from build123d import *

# Parameters (mm, degrees)
SKETCH1_W                    = 139.7
SKETCH1_H                    = 139.7
BOSS_EXTRUDE1_DEPTH          = 4.064
BOSS_EXTRUDE2_DEPTH          = 24.892
FILLET1_R                    = 4
FILLET2_R                    = 4
F_6_0_6_DIAMETER_HOLE1_D     = 6
F_6_0_6_DIAMETER_HOLE1_DEPTH = 18.75
F_6_0_6_DIAMETER_HOLE1_TIP   = 1.802581857


with BuildPart() as part:
    # Sketch1 → Boss-Extrude1 (new body)
    with BuildSketch(Plane(origin=(0, 0, 0), x_dir=(1, 0, 0), z_dir=(0, 1, 0))):
        Rectangle(SKETCH1_W, SKETCH1_H)
    extrude(amount=BOSS_EXTRUDE1_DEPTH)

    # Sketch2 → Boss-Extrude2 (add)
    with BuildSketch(Plane(origin=(0, 4.064, 0), x_dir=(1, 0, 0), z_dir=(0, 1, 0))):
        Polygon((27.6987, 69.85), (-27.6987, 69.85), (-27.6987, 56.261), (-48.5013, 56.261), (-48.5013, 69.85), (-69.85, 69.85), (-69.85, -69.85), (-48.5013, -69.85), (-48.5013, -56.261), (-27.6987, -56.261), (-27.6987, -69.85), (27.6987, -69.85), (27.6987, -56.261), (48.5013, -56.261), (48.5013, -69.85), (69.85, -69.85), (69.85, 69.85), (48.5013, 69.85), (48.5013, 56.261), (27.6987, 56.261), align=None)
    extrude(amount=BOSS_EXTRUDE2_DEPTH)

    # Fillet1
    fillet1_edges = [part.edges().sort_by_distance(p)[0] for p in [
        (48.5013, 16.51, 69.85),
        (48.5013, 16.51, -69.85),
        (48.5013, 16.51, -56.261),
        (27.6987, 16.51, -56.261),
        (27.6987, 16.51, -69.85),
        (-27.6987, 16.51, -69.85),
        (-27.6987, 16.51, -56.261),
        (-48.5013, 16.51, -56.261),
        (-48.5013, 16.51, -69.85),
        (-48.5013, 16.51, 69.85),
        (-48.5013, 16.51, 56.261),
        (-27.6987, 16.51, 56.261),
        (-27.6987, 16.51, 69.85),
        (27.6987, 16.51, 69.85),
        (27.6987, 16.51, 56.261),
        (48.5013, 16.51, 56.261),
        (69.85, 14.478, 69.85),
        (-69.85, 14.478, 69.85),
        (-69.85, 14.478, -69.85),
        (69.85, 14.478, -69.85),
    ]]
    fillet(fillet1_edges, radius=FILLET1_R)

    # Fillet2
    fillet2_edges = [part.edges().sort_by_distance(p)[0] for p in [
        (47.329727125, 28.956, -57.432572875),
        (28.870272875, 28.956, -57.432572875),
        (-28.870272875, 28.956, -57.432572875),
        (-47.329727125, 28.956, -57.432572875),
        (-47.329727125, 28.956, 57.432572875),
        (-28.870272875, 28.956, 57.432572875),
        (47.329727125, 28.956, 57.432572875),
        (28.870272875, 28.956, 57.432572875),
        (-59.17565, 28.956, -69.85),
        (0, 28.956, -69.85),
        (59.17565, 28.956, -69.85),
        (69.85, 28.956, 0),
        (59.17565, 28.956, 69.85),
        (48.5013, 28.956, -63.0555),
        (38.1, 28.956, -56.261),
        (27.6987, 28.956, -63.0555),
        (-27.6987, 28.956, -63.0555),
        (-38.1, 28.956, -56.261),
        (-48.5013, 28.956, -63.0555),
        (-69.85, 28.956, 0),
        (-59.17565, 28.956, 69.85),
        (-48.5013, 28.956, 63.0555),
        (-38.1, 28.956, 56.261),
        (-27.6987, 28.956, 63.0555),
        (0, 28.956, 69.85),
        (27.6987, 28.956, 63.0555),
        (38.1, 28.956, 56.261),
        (48.5013, 28.956, 63.0555),
        (68.678427125, 28.956, 68.678427125),
        (26.527127125, 28.956, 68.678427125),
        (49.672872875, 28.956, 68.678427125),
        (-26.527127125, 28.956, 68.678427125),
        (-49.672872875, 28.956, 68.678427125),
        (-68.678427125, 28.956, 68.678427125),
        (-68.678427125, 28.956, -68.678427125),
        (-49.672872875, 28.956, -68.678427125),
        (-26.527127125, 28.956, -68.678427125),
        (26.527127125, 28.956, -68.678427125),
        (49.672872875, 28.956, -68.678427125),
        (68.678427125, 28.956, -68.678427125),
    ]]
    fillet(fillet2_edges, radius=FILLET2_R)

    # Ø6.0 (6) Diameter Hole1
    with Locations(Plane(origin=(0, 4.064, 0), x_dir=(1, 0, 0), z_dir=(0, 1, 0))):
        with Locations((-38.1, 63.5), (38.1, 63.5), (38.1, -63.5), (-38.1, -63.5)):
            Hole(F_6_0_6_DIAMETER_HOLE1_D / 2, depth=F_6_0_6_DIAMETER_HOLE1_DEPTH)
            with Locations((0, 0, -(F_6_0_6_DIAMETER_HOLE1_DEPTH + F_6_0_6_DIAMETER_HOLE1_TIP / 2))):  # 118° drill point
                Cone(0, F_6_0_6_DIAMETER_HOLE1_D / 2, F_6_0_6_DIAMETER_HOLE1_TIP, mode=Mode.SUBTRACT)


solid = part.part
Read the model definition and answer for the solid it produces. Units are mm, in the model's axes. A direction names the side the tool comes from. Round coordinates to 2 decimals unless told otherwise and drop trailing zeros. Write each loop counter-clockwise with the first axis right and the second up, starting at its lowest first coordinate (ties: lowest second). Pieces come first, ordered by that corner, then holes.
1. Straight lines are drawn through the part: L1, parallel to Z at x = 38.1, y = 3.05; L2, parallel to X at y = 1.6, z = -63.5; L3, parallel to X at y = 7.75, z = -60. For each, find the intervals that lie inside material, in ascending order.
2. The part is cut by section A-A, the plane x = -38.1. Determine the outline of the cut face in (y, z), then the cut area to 3 significant figures.
3. Given pin 1 Ø6 at (x, y) = (-37.5, 5.5) entering from -Z; pin 2 Ø4 at (x, y) = (-35.5, 19.5) entering from -Z; pin 3 Ø4 at (x, z) = (33, -63) entering from +Y; pin 4 Ø14 at (x, y) = (-36, 17.5) entering from +Z, each flat-ended and moving along its own axis, determine where each tip first touches the part or whether it passes through.
4. The part is cut by section B-B, the plane z = 63.5. Determine the outline of the cut face in (x, y), then the cut area to 3 significant figures.
5. Determine the mould class of faces 4 (the face through (0.33, 27.75, -68.71)), 5 (the face through (-68.647, 12.653, 68.709)), 6 (the face through (49.64, 27.75, 63.02)) for opening direction X: pulls with the +X half, pulls with the -X half, needs draft (parallel to the pull), parting line crosses it, or undercut.
6. Which of the six approach directions +Z, -Z, +X, -X, +Y, -Y give full straight-line access (tool end or side, diameter ignored) to faces 1 (the face through (-1, 0, -1)), 2 (the face through (-49.64, 27.75, 63.09)), 3 (the face through (-38, 4.064, -60))?
Values:
1. L1: z = -69.85 to -66.5, -60.5 to 60.5, 66.5 to 69.85
1. L2: x = -69.85 to -41.1, -35.1 to 35.1, 41.1 to 69.85
1. L3: x = -69.85 to -48.49, -27.71 to 27.71, 48.49 to 69.85
2. outline: (0, -69.85) - (4.06, -69.85) - (4.06, -66.5) - (0, -66.5) - close; (0, -60.5) - (4.06, -60.5) - (4.06, -56.26) - (24.96, -56.26) arc R4 ccw to (28.96, -52.26) - (28.96, 52.26) arc R4 ccw to (24.96, 56.26) - (4.06, 56.26) - (4.06, 60.5) - (0, 60.5) - close; (0, 66.5) - (4.06, 66.5) - (4.06, 69.85) - (0, 69.85) - close
2. area: 3,310 mm2
3. pin 1: stops at z = -69.85
3. pin 2: stops at z = -56.26
3. pin 3: stops at y = 4.06
3. pin 4: stops at z = 57.31
4. outline: (-69.85, 0) - (-41.1, 0) - (-41.1, 4.06) - (-48.5, 4.06) - (-48.5, 24.96) arc R4 ccw to (-52.5, 28.96) - (-65.85, 28.96) arc R4 ccw to (-69.85, 24.96) - close; (-35.1, 0) - (35.1, 0) - (35.1, 4.06) - (27.7, 4.06) - (27.7, 24.96) arc R4 ccw to (23.7, 28.96) - (-23.7, 28.96) arc R4 ccw to (-27.7, 24.96) - (-27.7, 4.06) - (-35.1, 4.06) - close; (41.1, 0) - (69.85, 0) - (69.85, 24.96) arc R4 ccw to (65.85, 28.96) - (52.5, 28.96) arc R4 ccw to (48.5, 24.96) - (48.5, 4.06) - (41.1, 4.06) - close
4. area: 2,940 mm2
5. face 4: needs draft
5. face 5: pulls with the -X half
5. face 6: undercut
6. face 1: +Z, -Z, +X, -X, -Y
6. face 2: +Z, +Y
6. face 3: -Z, +Y
